The listing builds one solid part. Answer for the finished solid, in the listing's coordinates (mm). A direction names the side the tool comes from. Coordinates: 2 decimals unless noted, no trailing zeros. Loops run counter-clockwise (first coordinate to the right, second up) from the corner with the lowest first, then second, coordinate; pieces in that order, holes last. Notation, with made-up numbers: (2, -21.75) - (50, -21.75) arc R21 cw to (50, -12.75) - close; hole circle Ø8 at (20.5, 39.5). An arc over 180 degrees is marked (long way). Return JSON: item names as keys, results as strings. Group by question number.
1. Section D-D (y = -8.5) is taken. Write down the section's boundary in (x, z), and give its area (3 significant figures).
2. Section C-C (y = -5.25) is taken. Write down the section's boundary in (x, z), and give its area (3 significant figures).
3. The mould has two halves that part along Y. Classify faces 1 (the face through (15.72, -0.54, -12.19)), 2 (the face through (40.6, 0, 0)), 3 (the face through (-17, 7, 0)): pulls with the +Y half, pulls with the -Y half, needs draft (parallel to the pull), parting line crosses it, or undercut.
4. Each of these flat-tipped pins is pushed along its axis until it touches: P1, Ø1.8, axis at y = -8.5, z = 0, coming from the -X side; P2, Ø10, axis at y = -9, z = -7.5, coming from the +X side; P3, Ø5, axis at x = 14.5, y = 2.5, coming from the +Z side. Where does it stop, or does it pass through?
5. Find the intervals of material crossed by line 1 along Y through (x, z) = (-16.95, 0); line 2 along X through (y, z) = (6, 0); line 3 along X through (y, z) = (-11, 1.5), in increasing order.
6. Section B-B (z = 5.25) is taken. Write down the section's boundary in (x, y).
7. Which of the six approach directions +Z, -Z, +X, -X, +Y, -Y give full straight-line access (tool end or side, diameter ignored) to faces 4 (the face through (-31, 0, 0)), 5 (the face through (35, 15.5, 0)), 6 (the face through (35, 9.5, 0)), 7 (the face through (-20.232, 1.341, 3.233)), 8 (the face through (39, 1, 0))?
8. Section A-A (x = 35.5) is taken. Write down the section's boundary in (y, z), and give its area (3 significant figures).
```python
from build123d import *

# Parameters (mm, degrees)
SKETCH_3_W          = 4.5
SKETCH_3_H          = 7
SKETCH_3_W_2        = 31
SKETCH_3_H_2        = 12.2
SKETCH_3_W_3        = 9.5
SKETCH_3_H_3        = 2
SKETCH_3_W_4        = 2.5
SKETCH_3_H_4        = 1
SKETCH_4_R          = 1.5
CUT_EXTRUDE_1_DEPTH = 5
SKETCH_5_W          = 14
SKETCH_5_H          = 6
EXTRUDE_1_DEPTH     = 4.5


with BuildPart() as part:
    # Sketch 3 → Revolve 1 (revolve)
    with BuildSketch(Plane(origin=(0, 0, 0), x_dir=(1, 0, 0), z_dir=(0, 1, 0))):
        with Locations((35.85, -3.5)):
            Rectangle(SKETCH_3_W, SKETCH_3_H)
        with BuildLine():
            Line((33.6, 0), (32.6, 0))
            Line((32.6, 0), (32.6, -1))
            add(Edge.make_bspline(
                [(33.6, -1), (33.266666667, -1), (32.933333333, -1), (32.6, -1)],
                knots=[0, 0, 0, 0, 1, 1, 1, 1], degree=3))
            Line((33.6, -1), (33.6, 0))
        make_face()
        Polygon((32.6, 0), (31, 0), (31, -12.15), (32.6, -12.15), (32.6, -1), align=None)
        with Locations((15.5, -6.1)):
            Rectangle(SKETCH_3_W_2, SKETCH_3_H_2)
        Polygon((0, -12.2), (0, 0), (-19, 0), (-19, -3.5), (-19, -12.5), (0, -12.5), align=None)
        Polygon((-19, -3.5), (-19, 0), (-21.5, 0), (-21.5, -2), (-21.5, -3.5), align=None)
        with Locations((-26.25, -1)):
            Rectangle(SKETCH_3_W_3, SKETCH_3_H_3)
        with Locations((39.35, -0.5)):
            Rectangle(SKETCH_3_W_4, SKETCH_3_H_4)
    revolve(axis=Axis((-48.769222311, 0, 0), (1, 0, 0)))

    # Sketch 4 → Cut-Extrude 1 (cut)
    with BuildSketch(Plane.ZY.offset(19)):
        with Locations((0, 8.5)):
            Circle(SKETCH_4_R)
        with Locations((0, -8.5)):
            Circle(SKETCH_4_R)
    extrude(amount=-CUT_EXTRUDE_1_DEPTH, mode=Mode.SUBTRACT)

    # Sketch 5 → Extrude 1 (add)
    with BuildSketch(Plane(origin=(32.6, 0, 0), x_dir=(0, 0, -1), z_dir=(1, 0, 0))):
        with Locations((0, 12.5)):
            Rectangle(SKETCH_5_W, SKETCH_5_H)
    extrude(amount=EXTRUDE_1_DEPTH)


solid = part.part
```
The answers:
{
 "1": {"outline": "(-19, -9.17) - (0, -9.17) - (0, -8.75) - (31, -8.75) - (31, -8.68) - (32.6, -8.68) - (32.6, 8.68) - (31, 8.68) - (31, 8.75) - (0, 8.75) - (0, 9.17) - (-19, 9.17) - (-19, 1.5) - (-14, 1.5) - (-14, -1.5) - (-19, -1.5) - close", "area": "904 mm2"},
 "2": {"outline": "(-19, -11.34) - (0, -11.34) - (0, -11.01) - (31, -11.01) - (31, -10.96) - (32.6, -10.96) - (32.6, 10.96) - (31, 10.96) - (31, 11.01) - (0, 11.01) - (0, 11.34) - (-19, 11.34) - close; (33.6, -4.63) - (38.1, -4.63) - (38.1, 4.63) - (33.6, 4.63) - close", "area": "1,190 mm2"},
 "3": {"face 1": "parting line crosses it", "face 2": "needs draft", "face 3": "undercut"},
 "4": {"P1": "stops at x = -14", "P2": "stops at x = 38.1", "P3": "stops at z = 12.2"},
 "5": {"line 1": "y = -12.5 to -10, -7 to 7, 10 to 12.5", "line 2": "x = -19 to 32.6, 33.6 to 38.1", "line 3": "x = -19 to 32.6"},
 "6": {"outline": "(-19, -11.34) - (0, -11.34) - (0, -11.01) - (31, -11.01) - (31, -10.96) - (32.6, -10.96) - (32.6, 9.5) - (37.1, 9.5) - (37.1, 15.5) - (32.6, 15.5) - (32.6, 10.96) - (31, 10.96) - (31, 11.01) - (0, 11.01) - (0, 11.34) - (-19, 11.34) - close; (33.6, -4.63) - (38.1, -4.63) - (38.1, 4.63) - (33.6, 4.63) - close"},
 "7": {"face 4": "+Z, -Z, -X, +Y, -Y", "face 5": "+Z, -Z, +X, -X, +Y", "face 6": "+Z, -Z, +X", "face 7": "-X", "face 8": "+X"},
 "8": {"outline": "circle Ø14 at (0, 0); (9.5, -7) - (15.5, -7) - (15.5, 7) - (9.5, 7) - close", "area": "238 mm2"}
}
